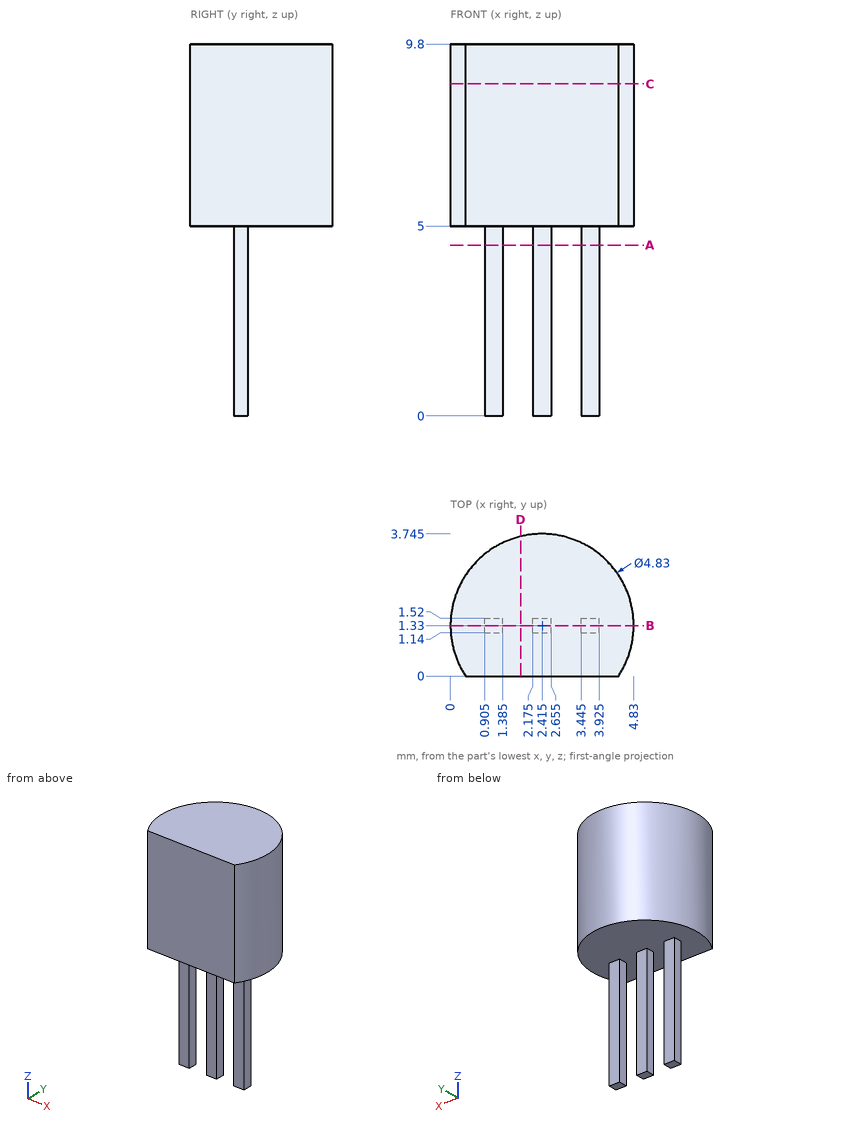
The drawing under review shows one solid part. Ordinate dimensions are in mm from its lowest x, y, z. Coordinates: 2 decimals unless noted, no trailing zeros. Order: outer loops, then holes, each group sorted by start corner. A loop starts at its lowest first (then second) coordinate and runs counter-clockwise, first axis right, second up. Notation, with made-up numbers: (-19.75, 59) -> (38.25, 59) arc R20 cw to (38.25, 95) -> close; hole circle Ø4 at (-16.5, 83). An arc over 180 degrees is marked (long way). Answer in a Markdown table with one row per item. Add a question column.
Item 1: To check wall thickness, follow probe 1 along X at (y, z) = (1.25, 3) (3 decimals); probe 2 along Z at (x, y) = (0.5, 0.2); probe 3 along Y at (x, z) = (1.05, 3.75). State the ranges of each line that lie inside material, in increasing order.
Item 2: Clearance check with flat-ended pins moving along their axes: pin 1 (0.5 mm diameter, centred on x = 3.5, z = 3.5, fed in from -Y); pin 2 (0.5 mm diameter, centred on x = 1, z = 3.5, fed in from +Y); pin 3 (1.5 mm diameter, centred on y = 1.5, z = 2, fed in from +X) (3 decimals). State where each tip first meets the part, or that it passes through.
Item 3: We need section C-C on z = 8.75. Write out the cut boundary in (x, y) (3 decimals), plus the area to 3 significant figures.
Item 4: We need section B-B on y = 1.33. Write out the cut boundary in (x, z) (3 decimals), plus the area to 3 significant figures.
Item 5: We need section D-D on x = 1.85. Write out the cut boundary in (y, z), plus the area to 3 significant figures.
Item 6: We need section A-A on z = 4.5. Write out the cut boundary in (x, y) (3 decimals).
Final values:
| question | item | result |
|---|---|---|
| 1 | probe 1 | x = 0.905 to 1.385, 2.175 to 2.655, 3.445 to 3.925 |
| 1 | probe 2 | z = 5 to 9.8 |
| 1 | probe 3 | y = 1.14 to 1.52 |
| 2 | pin 1 | stops at y = 1.14 |
| 2 | pin 2 | stops at y = 1.52 |
| 2 | pin 3 | stops at x = 3.925 |
| 3 | outline | (0.399, 0) -> (4.431, 0) arc R2.415 ccw (long way) to start |
| 3 | area | 15.2 mm2 |
| 4 | outline | (0, 5) -> (0.905, 5) -> (0.905, 0) -> (1.385, 0) -> (1.385, 5) -> (2.175, 5) -> (2.175, 0) -> (2.655, 0) -> (2.655, 5) -> (3.445, 5) -> (3.445, 0) -> (3.925, 0) -> (3.925, 5) -> (4.83, 5) -> (4.83, 9.8) -> (0, 9.8) -> close |
| 4 | area | 30.4 mm2 |
| 5 | outline | (0, 5) -> (3.68, 5) -> (3.68, 9.8) -> (0, 9.8) -> close |
| 5 | area | 17.7 mm2 |
| 6 | outline | (0.905, 1.14) -> (1.385, 1.14) -> (1.385, 1.52) -> (0.905, 1.52) -> close; (2.175, 1.14) -> (2.655, 1.14) -> (2.655, 1.52) -> (2.175, 1.52) -> close; (3.445, 1.14) -> (3.925, 1.14) -> (3.925, 1.52) -> (3.445, 1.52) -> close |
